Geometry: final body of the model. Coordinates: model frame, mm. A direction names the side the tool comes from. Coordinates: 2 decimals unless noted, no trailing zeros. Write each question's results on one line, items separated by ' | '. Start each with the question number.
from build123d import *

# Parameters (mm, degrees)
BOSS_EXTRUDE1_DEPTH         = 17.7165
FILLET1_R                   = 7.9375
F_3_4_16_TAPPED_HOLE1_D     = 17.4625
F_3_4_16_TAPPED_HOLE1_DEPTH = 15.875
F_3_4_16_TAPPED_HOLE2_D     = 17.4625
F_3_4_16_TAPPED_HOLE2_DEPTH = 15.875
SKETCH8_W                   = 25.4
SKETCH8_H                   = 22.86
CUT_EXTRUDE1_DEPTH          = 16.0655
FILLET2_R                   = 3.429
FILLET2_OF_MIRROR1_R        = 3.429
SKETCH10_R                  = 1.27
BOSS_EXTRUDE2_DEPTH         = 0.254
SKETCH15_W                  = 19.05
SKETCH15_H                  = 5.08
CUT_EXTRUDE2_DEPTH          = 1.905


with BuildPart() as part:
    # Sketch1 → Boss-Extrude1 (new, symmetric)
    with BuildSketch(Plane.XY):
        Polygon((47.625, 0), (0, 0), (0, 15.875), (47.625, 15.875), (47.625, 31.75), (-15.875, 31.75), (-15.875, -25.4), (31.75, -25.4), (31.75, -41.275), (-15.875, -41.275), (-15.875, -57.15), (47.625, -57.15), align=None)
    extrude(amount=BOSS_EXTRUDE1_DEPTH, both=True)

    # Fillet1
    fillet1_edges = [part.edges().sort_by_distance(p)[0] for p in [
        (31.75, -41.275, 0),
        (31.75, -25.4, 0),
        (0, 15.875, 0),
        (0, 0, 0),
    ]]
    fillet(fillet1_edges, radius=FILLET1_R - 0.0001)  # a hair under: the kernel refuses the full size

    # 3/4-16 Tapped Hole1
    with Locations(Plane.XZ.offset(57.15)):
        with Locations((15.875, 0)):
            Hole(F_3_4_16_TAPPED_HOLE1_D / 2, depth=F_3_4_16_TAPPED_HOLE1_DEPTH)

    # 3/4-16 Tapped Hole2
    with Locations(Plane(origin=(0, 31.75, 0), x_dir=(-1, 0, 0), z_dir=(0, 1, 0))):
        with Locations((-15.875, 0)):
            Hole(F_3_4_16_TAPPED_HOLE2_D / 2, depth=F_3_4_16_TAPPED_HOLE2_DEPTH)

    # Sketch8 → Cut-Extrude1 (cut)
    with BuildSketch(Plane.XY.offset(17.7165)):
        with Locations((15.875, -12.7)):
            Rectangle(SKETCH8_W, SKETCH8_H)
    cut_extrude1 = extrude(amount=-CUT_EXTRUDE1_DEPTH, mode=Mode.SUBTRACT)

    # Fillet2
    fillet2_edges = [part.edges().sort_by_distance(p)[0] for p in [
        (28.575, -1.27, 9.68375),
        (28.575, -24.13, 9.68375),
        (3.175, -24.13, 9.68375),
        (3.175, -1.27, 9.68375),
    ]]
    fillet(fillet2_edges, radius=FILLET2_R)

    # Mirror1: Cut-Extrude1 across plane
    add(cut_extrude1.mirror(Plane.XY), mode=Mode.SUBTRACT)

    # Fillet2 of Mirror1
    fillet2_of_mirror1_edges = [part.edges().sort_by_distance(p)[0] for p in [
        (28.575, -1.27, -9.68375),
        (28.575, -24.13, -9.68375),
        (3.175, -24.13, -9.68375),
        (3.175, -1.27, -9.68375),
    ]]
    fillet(fillet2_of_mirror1_edges, radius=FILLET2_OF_MIRROR1_R)

    # Sketch10 → Boss-Extrude2 (add)
    with BuildSketch(Plane.XY.offset(1.651)):
        with Locations(Location((15.875, -12.7, 0), (0, 0, 180))):
            Circle(SKETCH10_R)
    boss_extrude2 = extrude(amount=BOSS_EXTRUDE2_DEPTH)

    # Mirror2: Boss-Extrude2 across plane
    add(boss_extrude2.mirror(Plane.XY))

    # Sketch15 → Cut-Extrude2 (cut)
    with BuildSketch(Plane.XY.offset(17.7165)):
        with Locations((-6.35, -18.161)):
            Rectangle(SKETCH15_W, SKETCH15_H)
    extrude(amount=-CUT_EXTRUDE2_DEPTH, mode=Mode.SUBTRACT)


solid = part.part
Item 1: Section B-B, the plane z = 0. Count the separate pieces of the cut face and the enclosed holes in it, plus the area to 3 significant figures.
Item 2: Contact query for flat-ended pins moving along their axis: P1, Ø6, axis at x = 28.5, y = -15, coming from the +Z side; P2, Ø2, axis at x = 15.5, y = -12.5, coming from the +Z side (3 decimals); P3, Ø11.5, axis at x = 19, y = -13, coming from the -Z side (3 decimals). Output: stop coordinate, or through.
Item 3: Ray query, L1, parallel to Y at x = 9.5, z = 10.5 (3 decimals); L2, parallel to Y at x = -3, z = -7.5 (3 decimals); L3, parallel to Y at x = 36, z = -9.5 (3 decimals). Return the intervals inside material, ascending. Write a range as [from, to].
Item 4: Pull-direction query (X, two-part tool) for faces 6 (the cylindrical face through (2.387, 13.612, 0.248)), 7 (the cylindrical face through (4.206, -23.152, 9.571)), 8 (the flat face through (-15.875, -49, 0)); classes: released by +X, released by -X, zero draft, split by the parting line, or undercut.
Item 5: Set-up query: faces 1 (the cylindrical face through (7.547, -49.101, 2.623)), 2 (the flat face through (16, -24.13, 10)), 3 (the flat face through (28, 0, 0)), 4 (the flat face through (28.575, -13, -10)), 5 (the flat face through (4, -25.4, 0)). Return all of +Z, -Z, +X, -X, +Y, -Y with unobstructed straight access to the full face (end or side cutting, diameter ignored); none if empty.
Solutions:
1) separate pieces: 3 | enclosed holes: 0 | area: 3,630 mm²
2) P1: stops at z = 17.72 | P2: stops at z = 1.905 | P3: stops at z = -1.905
3) L1: y = [-57.15, -41.275], [-25.4, -24.13], [-1.27, 0], [15.875, 31.75] | L2: y = [-57.15, -41.275], [-25.4, 31.75] | L3: y = [-57.15, 0], [15.875, 31.75]
4) face 6: released by +X | face 7: undercut | face 8: released by -X
5) face 1: -Y | face 2: +Z | face 3: +Z, -Z, +X | face 4: -Z | face 5: +Z, -Z, -X
